Part model, mm, in its own coordinate system. Face numbers are marked on the shaded views. A direction names the side the tool comes from. Give positions to 0.01 mm unless a question says otherwise; leave off trailing zeros. Order: outer loops, then holes, each group sorted by start corner. A loop starts at its lowest first (then second) coordinate and runs counter-clockwise, first axis right, second up. Notation, with made-up numbers: M -34,73.25 L 6,73.25 A14 ccw 6,93.25 Z; hole C 56,31.5 d8. An arc over 180 degrees is marked long. One line per question, with ' | ' between items.
```python
from build123d import *

# Parameters (mm, degrees)
BOSS_EXTRUDE1_DEPTH = 1.875
SKETCH2_R           = 1
BOSS_EXTRUDE2_DEPTH = 30


with BuildPart() as part:
    # Sketch1 → Boss-Extrude1 (new body, symmetric)
    with BuildSketch(Plane(origin=(0, 0, 0), x_dir=(1, 0, 0), z_dir=(0, 1, 0))):
        Polygon((8.603650459, 4.727949427), (0.207300918, 9.814954576), (-8.396349541, 5.087005149), (-8.603650459, -4.727949427), (-0.207300918, -9.814954576), (8.396349541, -5.087005149), align=None)
    extrude(amount=BOSS_EXTRUDE1_DEPTH, both=True)

    # Sketch2 → Boss-Extrude2 (add)
    with BuildSketch(Plane(origin=(0, 1.875, 0), x_dir=(1, 0, 0), z_dir=(0, 1, 0))):
        Circle(SKETCH2_R)
    extrude(amount=BOSS_EXTRUDE2_DEPTH)

    # Sketch3 → Cut-Revolve1 (revolve, cut)
    with BuildSketch(Plane(origin=(0, 0, 0), x_dir=(0, 0, -1), z_dir=(1, 0, 0))):
        with BuildLine():
            Line((-7.638983711, -1.875), (-8.814954576, -1.875))
            ThreePointArc((-8.814954576, -1.875), (-9.522061357, -1.582106781), (-9.814954576, -0.875))
            Line((-9.814954576, -0.875), (-9.814954576, -0.236690097))
            Line((-9.814954576, -0.236690097), (-12.690091337, -2.588009386))
            Line((-12.690091337, -2.588009386), (-8.538791087, -3.391496898))
            Line((-8.538791087, -3.391496898), (-7.638983711, -1.875))
        make_face()
        with BuildLine():
            Line((-9.814954576, 0.342296512), (-9.814954576, 0.875))
            ThreePointArc((-9.814954576, 0.875), (-9.522061357, 1.582106781), (-8.814954576, 1.875))
            Line((-8.814954576, 1.875), (-7.819902103, 1.875))
            Line((-7.819902103, 1.875), (-11.754866647, 3.826938138))
            Line((-11.754866647, 3.826938138), (-9.814954576, 0.342296512))
        make_face()
    revolve(axis=Axis((0, 0, 0), (0, -1, 0)), mode=Mode.SUBTRACT)


solid = part.part
```
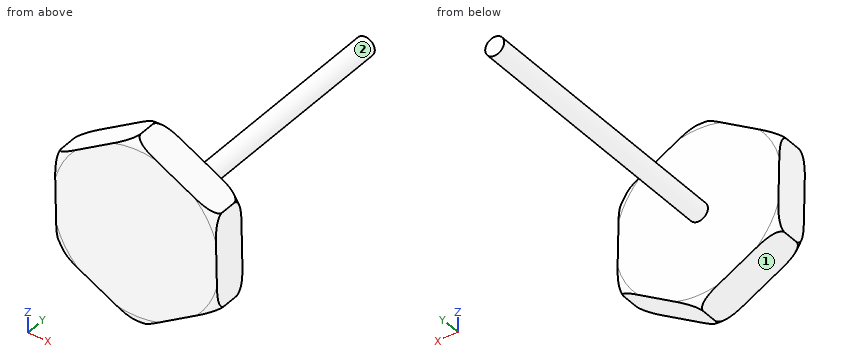
1. Probe L1, parallel to Y at x = 0.5, z = 5.75 (3 decimals); L2, parallel to Z at x = -0.5, y = 4.5; L3, parallel to X at y = 14, z = 0.25. List the from-to ranges inside material, lowest first. Write a range as from..to.
Worked out:
L1: y = -1.875..1.875 | L2: z = -0.87..0.87 | L3: x = -0.97..0.97
2. Slice it at C-C on x = -4.5. Give the cut face in (y, z) (3 decimals).
Worked out:
outline: M -1.875,-7.228 L 1.875,-7.228 L 1.875,7.214 L -1.875,7.214 Z
3. Slice it at B-B on y = 1.5. Give the cut face in (x, z).
Worked out:
outline: M -8.59,4.27 L -8.41,-4.63 A9.6 ccw -7.99,-5.31 L -0.2,-9.59 A9.6 ccw 0.6,-9.58 L 8.21,-4.97 A9.6 ccw 8.59,-4.27 L 8.41,4.63 A9.6 ccw 7.99,5.31 L 0.2,9.59 A9.6 ccw -0.6,9.58 L -8.21,4.97 A9.6 ccw Z
4. Tool access for the marked faces 1 and 2: list every direction of +Z, -Z, +X, -X, +Y, -Y with a clear straight run to the whole face (end or side of a thin tool).
Worked out:
face 1: -Z, -X, +Y, -Y | face 2: +Y
5. Slice it at D-D on y = 7. Give the cut face in (x, z), then the cut area to 3 significant figures.
Worked out:
outline: C 0,0 d2 | area: 3.14 mm2
6. Drop flat-ended pins along their axis: pin 1 (4 mm diameter, centred on y = 26.5, z = -2, fed in from -X); pin 2 (2 mm diameter, centred on x = -5, z = -1, fed in from +Y) (3 decimals); pin 3 (1 mm diameter, centred on x = -2, y = 14.5, fed in from -Z); pin 4 (1 mm diameter, centred on y = 1.5, z = 2, fed in from -X). Give the stop position or say it passes through.
Worked out:
pin 1: stops at x = -1 | pin 2: stops at y = 1.875 | pin 3: passes through | pin 4: stops at x = -8.56
7. Slice it at A-A on z = 0. Give the cut face in (x, y) (3 decimals).
Worked out:
outline: M -8.504,-1.875 L 8.504,-1.875 L 8.504,1.875 L 1,1.875 L 1,31.875 L -1,31.875 L -1,1.875 L -8.504,1.875 Z
